from build123d import *

# Parameters (mm, degrees)
F2_DEPTH  = 1910
F7_DEPTH  = 1120
F9_DEPTH  = 2000
F11_DEPTH = 700


# Not quite as in the source:
# - ends of sketch curves that miss each other by under 0.0002 mm in the source are joined


with BuildPart() as f2:
    # F1 (on Front) → F2 (new body)
    with BuildSketch(Plane.XZ):
        with BuildLine():
            Line((7.5, 37.974085065), (7.5, 40))
            Line((7.5, 40), (-15, 40))
            Line((-15, 40), (-15, 37))
            Line((-15, 37), (-15, 31))
            Line((-15, 31), (-15, 29))
            Line((-15, 29), (-15, 26))
            Line((-15, 26), (-15, 24))
            Line((-15, 24), (-13, 24))
            Line((-13, 24), (-11, 24))
            Line((-11, 24), (-11, 26))
            Line((-11, 26), (-9, 26))
            Line((-9, 26), (-9, 20))
            Line((-9, 20), (-11, 20))
            Line((-11, 20), (-11, 22))
            Line((-11, 22), (-15, 22))
            Line((-15, 22), (-15, 18))
            Line((-15, 18), (-15, 7.7))
            Line((-15, 7.7), (-13, 7.7))
            Line((-13, 7.7), (-13, 11.4920835048))
            Line((-13, 11.4920835048), (-7, 11.4920835048))
            Line((-7, 11.4920835048), (-7, 3.7))
            Line((-7, 3.7), (-11, 3.7))
            Line((-11, 3.7), (-11, 5.7))
            Line((-11, 5.7), (-15, 5.7))
            Line((-15, 5.7), (-15, 3))
            Line((-15, 3), (-15, 0))
            Line((-15, 0), (-13, 0))
            Line((-13, 0), (-12, 0))
            Line((-12, 0), (-5, 0))
            Line((-5, 0), (-5, 13.4920835048))
            Line((-5, 13.4920835048), (-7, 13.4920835048))
            Line((-7, 13.4920835048), (-9.1588944197, 13.4920835048))
            Line((-9.1588944197, 13.4920835048), (-9.1588944197, 15.4920835048))
            Line((-9.1588944197, 15.4920835048), (1.5, 20))
            Line((1.5, 20), (10.8411055803, 15.4920835048))
            Line((10.8411055803, 15.4920835048), (10.8411055803, 13.4920835048))
            Line((10.8411055803, 13.4920835048), (8, 13.4920835048))
            Line((8, 13.4920835048), (8, 0))
            Line((8, 0), (17, 0))
            Line((17, 0), (17, 40))
            Line((17, 40), (8.5, 40))
            Line((8.5, 40), (8.5, 37.974085065))
            ThreePointArc((8.5, 37.974085065), (11.5604089792, 36.6859489396), (13.3185590744, 33.8691589154))
            Line((13.3185590744, 33.8691589154), (13.4318527537, 31.7073867348))
            ThreePointArc((13.4318527537, 31.7073867348), (4.0126863822, 28.7323088758), (7.5, 37.974085065))
        make_face()
        Polygon((-8.3634709733, 18), (-11.1588944197, 16.817744602), (-11.1588944197, 15.4920835048), (-11.1588944197, 13.4920835048), (-13, 13.4920835048), (-13, 18), align=None, mode=Mode.SUBTRACT)
        with BuildLine():
            Line((-13, 34), (-13, 37.9999987781))
            Line((-13, 37.9999987781), (2.9081163149, 37.9999987781))
            ThreePointArc((2.9081163149, 37.9999987781), (3.810445381, 26.2974906682), (15, 29.8410427327))
            Line((15, 29.8410427327), (15, 2))
            Line((15, 2), (10, 2))
            Line((10, 2), (10, 12))
            Line((10, 12), (12.8411055803, 12))
            Line((12.8411055803, 12), (12.8411055803, 16.7476188273))
            Line((12.8411055803, 16.7476188273), (1.5543358685, 22.194491783))
            Line((1.5543358685, 22.194491783), (-7, 18.5766464184))
            Line((-7, 18.5766464184), (-7, 28))
            Line((-7, 28), (-13, 28))
            Line((-13, 28), (-13, 34))
        make_face(mode=Mode.SUBTRACT)
        with BuildLine():
            Line((13.0918836851, 37.9999987781), (13.1020709306, 37.9999987781))
            Line((13.1020709306, 37.9999987781), (13.1025921338, 37.9900536295))
            ThreePointArc((13.1025921338, 37.9900536295), (13.0972403349, 37.9950288154), (13.0918836851, 37.9999987781))
        make_face(mode=Mode.SUBTRACT)
    extrude(amount=-F2_DEPTH)

    # F6 (on Front) → F7 (join)
    with BuildSketch(Plane.XZ):
        with BuildLine():
            Line((8.5, 37.3712719703), (8.5, 40))
            Line((8.5, 40), (8.5, 41))
            Line((8.5, 41), (-198.8, 41))
            Line((-198.8, 41), (-198.8, 40))
            Line((-198.8, 40), (-25.5, 40))
            Line((-25.5, 40), (-15, 40))
            Line((-15, 40), (7.5, 40))
            Line((7.5, 40), (7.5, 37.3712723193))
            ThreePointArc((7.5, 37.3712723193), (7.9999999822, 27.6162403216), (8.5, 37.3712719703))
        make_face()
    extrude(amount=-F7_DEPTH)

    # F8 (on face) → F9 (cut)
    with BuildSketch(Plane.XZ):
        with BuildLine():
            Line((-15, 3), (-15, 0))
            Line((-15, 0), (-13, 0))
            Line((-13, 0), (-12, 0))
            Line((-12, 0), (-5, 0))
            Line((-5, 0), (-5, 13.4920835048))
            Line((-5, 13.4920835048), (-7, 13.4920835048))
            Line((-7, 13.4920835048), (-9.1588944197, 13.4920835048))
            Line((-9.1588944197, 13.4920835048), (-9.1588944197, 15.4920835048))
            Line((-9.1588944197, 15.4920835048), (1.5, 20))
            Line((1.5, 20), (10.8411055803, 15.4920835048))
            Line((10.8411055803, 15.4920835048), (10.8411055803, 13.4920835048))
            Line((10.8411055803, 13.4920835048), (8, 13.4920835048))
            Line((8, 13.4920835048), (8, 0))
            Line((8, 0), (17, 0))
            Line((17, 0), (17, 40))
            Line((17, 40), (8.5, 40))
            Line((8.5, 40), (8.5, 37.974085065))
            ThreePointArc((8.5, 37.974085065), (11.5604089792, 36.6859489396), (13.3185590744, 33.8691589154))
            Line((13.3185590744, 33.8691589154), (13.4318527537, 31.7073867348))
            ThreePointArc((13.4318527537, 31.7073867348), (4.0126863822, 28.7323088758), (7.5, 37.974085065))
            Line((7.5, 37.974085065), (7.5, 40))
            Line((7.5, 40), (-15, 40))
            Line((-15, 40), (-15, 31))
            Line((-15, 31), (-15, 29))
            Line((-15, 29), (-15, 24))
            Line((-15, 24), (-13, 24))
            Line((-13, 24), (-11, 24))
            Line((-11, 24), (-11, 26))
            Line((-11, 26), (-9, 26))
            Line((-9, 26), (-9, 20))
            Line((-9, 20), (-11, 20))
            Line((-11, 20), (-11, 22))
            Line((-11, 22), (-15, 22))
            Line((-15, 22), (-15, 18))
            Line((-15, 18), (-15, 7.7))
            Line((-15, 7.7), (-13, 7.7))
            Line((-13, 7.7), (-13, 11.4920835048))
            Line((-13, 11.4920835048), (-7, 11.4920835048))
            Line((-7, 11.4920835048), (-7, 3.7))
            Line((-7, 3.7), (-11, 3.7))
            Line((-11, 3.7), (-11, 5.7))
            Line((-11, 5.7), (-15, 5.7))
            Line((-15, 5.7), (-15, 3))
        make_face()
        Polygon((-13, 18), (-8.3634709733, 18), (-11.1588944197, 16.817744602), (-11.1588944197, 15.4920835048), (-11.1588944197, 13.4920835048), (-13, 13.4920835048), align=None, mode=Mode.SUBTRACT)
        with BuildLine():
            Line((12.8411055803, 12), (12.8411055803, 16.7476188273))
            Line((12.8411055803, 16.7476188273), (1.5543358685, 22.194491783))
            Line((1.5543358685, 22.194491783), (-7, 18.5766464184))
            Line((-7, 18.5766464184), (-7, 28))
            Line((-7, 28), (-13, 28))
            Line((-13, 28), (-13, 34))
            Line((-13, 34), (-13, 37.9999987781))
            Line((-13, 37.9999987781), (2.9081163149, 37.9999987781))
            ThreePointArc((2.9081163149, 37.9999987781), (3.810445381, 26.2974906682), (15, 29.8410427327))
            Line((15, 29.8410427327), (15, 2))
            Line((15, 2), (10, 2))
            Line((10, 2), (10, 12))
            Line((10, 12), (12.8411055803, 12))
        make_face(mode=Mode.SUBTRACT)
    extrude(amount=-F9_DEPTH, mode=Mode.SUBTRACT)

    # F10 (on face) → F11 (join)
    with BuildSketch(Plane.XZ):
        with BuildLine():
            Line((-49.096, 40), (-26.596, 40))
            Line((-26.596, 40), (-26.596, 37.9675733099))
            ThreePointArc((-26.596, 37.9675733099), (-25.951759356, 27.0133522571), (-25.5, 37.9771982231))
            Line((-25.5, 37.9771982231), (-25.5, 41))
            Line((-25.5, 41), (-198.8, 41))
            Line((-198.8, 41), (-198.8, 40))
            Line((-198.8, 40), (-49.096, 40))
        make_face()
    extrude(amount=F11_DEPTH)

    # F12: F2 across face


with BuildPart() as f2_1:
    add(f2.part)
    add(f2.part.mirror(Plane(origin=(-198.8, 210, 40.5), x_dir=(0, -1, 0), z_dir=(-1, 0, 0))))


solid = f2_1.part
Can you work these out from the model? Positions are in its coordinate system, mm. Round coordinates to 2 decimals unless told otherwise and drop trailing zeros. Write each loop counter-clockwise with the first axis right and the second up, starting at its lowest first coordinate (ties: lowest second). Pieces come first, ordered by that corner, then holes. Notation, with made-up numbers: M 6.25,37 L 40.25,37 A4 ccw 40.25,41 Z; hole C 50,-38.75 d6. An arc over 180 degrees is marked long. Use a Markdown table: item, result.
Item 1: If I drill on line 1 along X through (y, z) = (178.5, 33.5); line 2 along X through (y, z) = (265.5, 32.25); line 3 along Z through (x, y) = (-197, 872), over which ranges is the centre line in solid material (lowest first)? Write a range as [from, to].
Found:
| item | result |
|---|---|
| line 1 | x = [-410.39, -400.81], [3.21, 12.79] |
| line 2 | x = [-410.48, -400.72], [3.12, 12.88] |
| line 3 | z = [40, 41] |
Item 2: I want a section at C-C (x = -163). List the corners of the cut face in (y, z) for me, and give its area (3 significant figures).
Found:
| item | result |
|---|---|
| outline | M -700,40 L 1120,40 L 1120,41 L -700,41 Z |
| area | 1,820 mm2 |
Item 3: For pin 1 Ø5.5 at (x, z) = (-25, 30.5) entering from +Y; pin 2 Ø1 at (y, z) = (448, 31) entering from +X; pin 3 Ø8 at (y, z) = (-434.5, 30) entering from -X, each with a flat end and sliding along its axis, tell me the tip position at first contact or that it passes through.
Found:
| item | result |
|---|---|
| pin 1 | stops at y = 0 |
| pin 2 | stops at x = 12.79 |
| pin 3 | stops at x = -377.09 |
Item 4: I want a section at A-A (y = -24.5). List the corners of the cut face in (x, z) for me, and give its area (3 significant figures).
Found:
| item | result |
|---|---|
| outline | M -372.1,37.98 A5.49 ccw long -371,37.97 L -371,40 L -26.6,40 L -26.6,37.97 A5.49 ccw long -25.5,37.98 L -25.5,41 L -372.1,41 Z |
| area | 541 mm2 |
Item 5: I want a section at B-B (z = 34.5). List the corners of the cut face in (x, y) for me, and give its area (3 significant figures).
Found:
| item | result |
|---|---|
| outline | M -410.07,0 L -401.13,0 L -401.13,1120 L -410.07,1120 Z; M -376.72,-700 L -366.48,-700 L -366.48,0 L -376.72,0 Z; M -31.12,-700 L -20.88,-700 L -20.88,0 L -31.12,0 Z; M 3.53,0 L 12.47,0 L 12.47,1120 L 3.53,1120 Z |
| area | 34,300 mm2 |
